CAD build for the part. Positions are in the model's coordinates, mm. A direction names the side the tool comes from. Give positions to 0.01 mm unless a question says otherwise; leave off trailing zeros. Write each loop counter-clockwise with the first axis right and the second up, starting at its lowest first coordinate (ties: lowest second). Pieces come first, ordered by that corner, then holes. Notation, with made-up numbers: (8.25, 0) - (46.25, 0) arc R31 ccw to (46.25, 32) - close; hole circle Ø11 at (-38, 27.5). An arc over 180 degrees is marked (long way). Answer as a JSON object with one key per item and string values.
from build123d import *
from build123d.topology import SkipClean

# Parameters (mm, degrees)
CROQUIS1_R              = 1.5
SALIENTE_EXTRUIR1_DEPTH = 15
CROQUIS2_R              = 2.5
CORTAR_EXTRUIR1_DEPTH   = 20
CORTAR_EXTRUIR2_START   = -22
CORTAR_EXTRUIR2_DEPTH   = 22


with BuildPart() as part:
    # Croquis1 → Saliente-Extruir1 (new body)
    with BuildSketch(Plane.XY):
        with BuildLine():
            Line((11.25, 17.1), (11.25, 11.1))
            Line((11.25, 11.1), (23.75, 11.1))
            Line((23.75, 11.1), (23.75, 5.1))
            Line((23.75, 5.1), (11.25, 5.1))
            Line((11.25, 5.1), (11.25, -0.9))
            Line((11.25, -0.9), (5.75, -0.9))
            ThreePointArc((5.75, -0.9), (0.800252532, 1.150252532), (-1.25, 6.1))
            Line((-1.25, 6.1), (-1.25, 10.1))
            ThreePointArc((-1.25, 10.1), (0.800252532, 15.049747468), (5.75, 17.1))
            Line((5.75, 17.1), (11.25, 17.1))
        make_face()
        with Locations((3.75, 8.1)):
            Circle(CROQUIS1_R, mode=Mode.SUBTRACT)
    extrude(amount=SALIENTE_EXTRUIR1_DEPTH)

    # Croquis2 → Cortar-Extruir1 (cut)
    with BuildSketch(Plane(origin=(0, 0, 0), x_dir=(1, 0, 0), z_dir=(0, 1, 0))):
        with Locations(Location((17.5, -7.5, 0), (0, 0, 90))):
            Circle(CROQUIS2_R)
        with BuildLine():
            Line((17.5, -1.25), (11.25, 0))
            Line((11.25, 0), (11.126279301, 1.868603497))
            Line((11.126279301, 1.868603497), (29.663453957, 1.868603497))
            Line((29.663453957, 1.868603497), (29.663453957, -17.961269996))
            Line((29.663453957, -17.961269996), (11.25, -17.961269996))
            Line((11.25, -17.961269996), (11.25, -15))
            Line((11.25, -15), (17.5, -13.75))
            ThreePointArc((17.5, -13.75), (23.75, -7.5), (17.5, -1.25))
        make_face()
    extrude(amount=CORTAR_EXTRUIR1_DEPTH, mode=Mode.SUBTRACT)

    # Croquis3 → Cortar-Extruir2 (cut)
    with SkipClean():  # the faces are left unmerged after this step: merging them gives an invalid solid
        with BuildSketch(Plane(origin=(0, 17.1, 0), x_dir=(1, 0, 0), z_dir=(0, 1, 0)).offset(CORTAR_EXTRUIR2_START)):
            with BuildLine():
                Line((-4.130088798, -10), (11.25, -10))
                Line((11.25, -10), (11.985294118, -10.441176471))
                ThreePointArc((11.985294118, -10.441176471), (14.284401529, -12.859330786), (17.5, -13.75))
                Line((17.5, -13.75), (17.5, -15.581395259))
                Line((17.5, -15.581395259), (-4.130088798, -15.581395259))
                Line((-4.130088798, -15.581395259), (-4.130088798, -10))
            make_face()
            with BuildLine():
                Line((-3.464792336, -5), (11.25, -5))
                Line((11.25, -5), (11.985294118, -4.558823529))
                ThreePointArc((11.985294118, -4.558823529), (14.284401529, -2.140669214), (17.5, -1.25))
                Line((17.5, -1.25), (17.5, 1.677177667))
                Line((17.5, 1.677177667), (-3.464792336, 1.677177667))
                Line((-3.464792336, 1.677177667), (-3.464792336, -5))
            make_face()
        extrude(amount=CORTAR_EXTRUIR2_DEPTH, mode=Mode.SUBTRACT)


solid = part.part
(1) Probe L1, parallel to Y at x = 14.25, z = 8.75; L2, parallel to X at y = 9.75, z = 7.5; L3, parallel to Y at x = 3.75, z = 8.6. List the from-to ranges inside material, lowest first. Write a range as [from, to].
Answer key:
{"L1": "y = [5.1, 11.1]", "L2": "x = [-1.25, 15], [20, 23.75]", "L3": "y = [-0.61, 6.6], [9.6, 16.81]"}
(2) Saw through at B-B, the plane y = 8.1. Give the cut face in (x, z), and give its area (3 significant figures).
Answer key:
{"outline": "(-1.25, 5) - (2.25, 5) - (2.25, 10) - (-1.25, 10) - close; (5.25, 5) - (11.25, 5) - (11.99, 4.56) arc R6.25 ccw (long way) to (11.99, 10.44) - (11.25, 10) - (5.25, 10) - close; hole circle Ø5 at (17.5, 7.5)", "area": "152 mm²"}
(3) Pull direction Z, two halves, no side cores. Call faces 1 (the face through (17.4, 11.1, 10.2)), 2 (the face through (6, 8, 10)), 3 (the face through (6, 8, 5)), 4 (the face through (19.94, 8.06, 8.04)): pulls with the +Z half, pulls with the -Z half, needs draft (parallel to the pull), parting line crosses it, or undercut.
Answer key:
{"face 1": "needs draft", "face 2": "pulls with the +Z half", "face 3": "pulls with the -Z half", "face 4": "undercut"}
(4) Saw through at D-D, the plane z = 9. Give the cut face in (x, y), and give its area (3 significant figures).
Answer key:
{"outline": "(-1.25, 6.1) arc R7 ccw to (5.75, -0.9) - (11.25, -0.9) - (11.25, 5.1) - (15.5, 5.1) - (15.5, 11.1) - (11.25, 11.1) - (11.25, 17.1) - (5.75, 17.1) arc R7 ccw to (-1.25, 10.1) - close; (19.5, 5.1) - (23.57, 5.1) - (23.57, 11.1) - (19.5, 11.1) - close; hole circle Ø3 at (3.75, 8.1)", "area": "247 mm²"}
(5) Flat gauge pins, fed straight in: P1, Ø2.5, axis at y = 2.5, z = 8.5, coming from the +X side; P2, Ø6, axis at x = 6.5, y = 6.5, coming from the +Z side; P3, Ø4, axis at x = 6.5, y = 7, coming from the -Z side. Where does each tip first touch, or does it go through?
Answer key:
{"P1": "stops at x = 11.25", "P2": "stops at z = 10", "P3": "stops at z = 5"}
(6) 3-axis set-ups, long thin cutter, end or side, ignore diameter. For faces 5 (the face through (17.6, 5.1, 10.2)), 6 (the face through (11.25, 14, 7)), 7 (the face through (4.556, 9.365, 7.465)): which of +Z, -Z, +X, -X, +Y, -Y reach the whole face in a straight line?
Answer key:
{"face 5": "+Z, -Z, +X, -Y", "face 6": "+Z, -Z, +X, +Y", "face 7": "+Z, -Z"}
(7) Saw through at C-C, the plane x = 19.25. Give the cut face in (y, z).
Answer key:
{"outline": "(5.1, 1.5) - (11.1, 1.5) - (11.1, 5.71) - (5.1, 5.71) - close; (5.1, 9.29) - (11.1, 9.29) - (11.1, 13.5) - (5.1, 13.5) - close"}
(8) Saw through at A-A, the plane z = 7.5. Give the cut face in (x, y), and give its area (3 significant figures).
Answer key:
{"outline": "(-1.25, 6.1) arc R7 ccw to (5.75, -0.9) - (11.25, -0.9) - (11.25, 5.1) - (15, 5.1) - (15, 11.1) - (11.25, 11.1) - (11.25, 17.1) - (5.75, 17.1) arc R7 ccw to (-1.25, 10.1) - close; (20, 5.1) - (23.75, 5.1) - (23.75, 11.1) - (20, 11.1) - close; hole circle Ø3 at (3.75, 8.1)", "area": "242 mm²"}
